from build123d import *

# Parameters (mm, degrees)
TAP_DRILL_FOR_M3_HELICOIL1_D     = 3.15
TAP_DRILL_FOR_M3_HELICOIL1_DEPTH = 10
TAP_DRILL_FOR_M3_HELICOIL1_TIP   = 0.946355475
CUT_EXTRUDE3_REACH               = 22.213
SKETCH2_R                        = 1.25


with BuildPart() as part:
    # Sketch1 → Revolve1 (revolve)
    with BuildSketch(Plane(origin=(0, 0, 0), x_dir=(0, 0, -1), z_dir=(1, 0, 0))):
        Polygon((0, 3), (-8.4, 3), (-8.4, 6), (-4.8, 6), (-4.8, 13), (0, 13), align=None)
    revolve(axis=Axis((0, 0, 6.17319531), (0, 0, 1)))

    # Tap Drill for M3 Helicoil1
    with Locations(Plane(origin=(0, -9.5, 4.8), x_dir=(0, 1, 0), z_dir=(0, 0, 1))):
        with Locations((0, 0), (4.75, -8.227241336), (14.25, -8.227241336), (19, 0), (14.25, 8.227241336), (4.75, 8.227241336)):
            Hole(TAP_DRILL_FOR_M3_HELICOIL1_D / 2, depth=TAP_DRILL_FOR_M3_HELICOIL1_DEPTH)
            with Locations((0, 0, -(TAP_DRILL_FOR_M3_HELICOIL1_DEPTH + TAP_DRILL_FOR_M3_HELICOIL1_TIP / 2))):  # 118° drill point
                Cone(0, TAP_DRILL_FOR_M3_HELICOIL1_D / 2, TAP_DRILL_FOR_M3_HELICOIL1_TIP, mode=Mode.SUBTRACT)

    # Sketch2 → Cut-Extrude3 (cut, up to next)
    with BuildSketch(Plane(origin=(0, 0, 0), x_dir=(0, 0, -1), z_dir=(1, 0, 0)), mode=Mode.PRIVATE) as cut_extrude3_sk1:
        with Locations((-2.4, 0)):
            Circle(SKETCH2_R)
    cut_extrude3_tool1 = extrude(cut_extrude3_sk1.sketch, amount=-CUT_EXTRUDE3_REACH, mode=Mode.PRIVATE) & part.part
    # Sketch2 → Cut-Extrude3 (cut, up to next)
    with BuildSketch(Plane(origin=(0, 0, 0), x_dir=(0, 0, -1), z_dir=(1, 0, 0)), mode=Mode.PRIVATE) as cut_extrude3_sk2:
        with Locations((-6.6, 0)):
            Circle(SKETCH2_R)
    cut_extrude3_tool2 = extrude(cut_extrude3_sk2.sketch, amount=-CUT_EXTRUDE3_REACH, mode=Mode.PRIVATE) & part.part
    add(cut_extrude3_tool1.solids().sort_by_distance((0, 0, 2.4))[0], mode=Mode.SUBTRACT)
    add(cut_extrude3_tool2.solids().sort_by_distance((0, 0, 6.6))[0], mode=Mode.SUBTRACT)


solid = part.part
Read the model definition and answer for the solid it produces. Units are mm, in the model's axes. A direction names the side the tool comes from. Coordinates: 2 decimals unless noted, no trailing zeros. Write each loop counter-clockwise with the first axis right and the second up, starting at its lowest first coordinate (ties: lowest second). Pieces come first, ordered by that corner, then holes. Notation, with made-up numbers: (-12, 75.5) -> (-2, 75.5) arc R10 cw to (-2, 93.5) -> close; hole circle Ø11 at (61, 57.5). An arc over 180 degrees is marked (long way). Return JSON: item names as keys, results as strings.
(1) The part is cut by section D-D on z = 2.4. Give the vertices of the cut face in (x, y) (3 decimals).
Answers below:
{"outline": "(-12.94, -1.25) arc R13 ccw (long way) to (-12.94, 1.25) -> (-2.727, 1.25) arc R3 cw (long way) to (-2.727, -1.25) -> close; hole circle Ø3.15 at (-8.227, -4.75); hole circle Ø3.15 at (-8.227, 4.75); hole circle Ø3.15 at (0, -9.5); hole circle Ø3.15 at (0, 9.5); hole circle Ø3.15 at (8.227, -4.75); hole circle Ø3.15 at (8.227, 4.75)"}
(2) For a pull along X with two mould halves and no side action, classify faces 1 (the cylindrical face through (5.857, -1.301, 6.575)), 2 (the cylindrical face through (-9.29, -3.59, 2.37)), 3 (the flat face through (1, 3, 8.4)), 4 (the cylindrical face through (7.16, -3.59, 2.37)) as pulls with the +X half, pulls with the -X half, needs draft (parallel to the pull), parting line crosses it, or undercut.
Answers below:
{"face 1": "parting line crosses it", "face 2": "undercut", "face 3": "needs draft", "face 4": "undercut"}
(3) The part is cut by section C-C on y = -10. Give the vertices of the cut face in (x, z).
Answers below:
{"outline": "(-8.31, 0) -> (-1.49, 0) -> (-1.49, 4.8) -> (-8.31, 4.8) -> close; (1.49, 0) -> (8.31, 0) -> (8.31, 4.8) -> (1.49, 4.8) -> close"}
(4) Each of these flat-tipped pins is pushed along its axis until it touches: P1, Ø5, axis at x = 8.23, y = 4.75, coming from the +Z side; P2, Ø5, axis at y = 5.5, z = 2, coming from the +X side; P3, Ø3, axis at x = -8.23, y = 4.75, coming from the +Z side; P4, Ø4, axis at x = -7.5, z = 2, coming from the -Y side. Where does it stop, or does it pass through?
Answers below:
{"P1": "z = 4.8", "P2": "x = 12.65", "P3": "through", "P4": "y = -11.78"}
(5) Consider line 1 along Y through (x, z) = (7.25, 2.5); line 2 along Y through (x, z) = (0, 6.5); line 3 along X through (y, z) = (-3.5, 1.75). Determine where each line is inside the solid, lowest interval first. Write a range as from..to.
Answers below:
{"line 1": "-10.79..-5.99, -3.51..3.51, 5.99..10.79", "line 2": "-6..-3, 3..6", "line 3": "-12.52..-9.19, -7.27..7.27, 9.19..12.52"}
(6) Which of the six approach directions +Z, -Z, +X, -X, +Y, -Y give full straight-line access (tool end or side, diameter ignored) to faces 5 (the cylindrical face through (-9.79, 4.96, 2.37)), 6 (the cylindrical face through (-4.34, 1.24, 6.76)), 7 (the flat face through (3, -6, 4.8))?
Answers below:
{"face 5": "+Z, -Z", "face 6": "-X", "face 7": "+Z"}
(7) The part is cut by section B-B on y = -3.5. Give the vertices of the cut face in (x, z), then the cut area to 3 significant figures.
Answers below:
{"outline": "(-12.52, 0) -> (-9.19, 0) -> (-9.19, 4.8) -> (-12.52, 4.8) -> close; (-7.27, 0) -> (7.27, 0) -> (7.27, 4.8) -> (4.87, 4.8) -> (4.87, 8.4) -> (-4.87, 8.4) -> (-4.87, 4.8) -> (-7.27, 4.8) -> close; (9.19, 0) -> (12.52, 0) -> (12.52, 4.8) -> (9.19, 4.8) -> close", "area": "137 mm^2"}
(8) The part is cut by section A-A on x = 0. Give the vertices of the cut face in (y, z) (3 decimals), then the cut area to 3 significant figures.
Answers below:
{"outline": "(-13, 0) -> (-11.075, 0) -> (-11.075, 4.8) -> (-13, 4.8) -> close; (-7.925, 0) -> (-3, 0) -> (-3, 8.4) -> (-6, 8.4) -> (-6, 4.8) -> (-7.925, 4.8) -> close; (3, 0) -> (7.925, 0) -> (7.925, 4.8) -> (6, 4.8) -> (6, 8.4) -> (3, 8.4) -> close; (11.075, 0) -> (13, 0) -> (13, 4.8) -> (11.075, 4.8) -> close", "area": "87.4 mm^2"}
